from build123d import *

# Parameters (mm, degrees)
BOSS_EXTRUDE1_DEPTH = 5
SKETCH4_R           = 1.75
CUT_EXTRUDE1_DEPTH  = 5
CUT_EXTRUDE2_DEPTH  = 5
SKETCH6_R           = 1.75
BOSS_EXTRUDE2_DEPTH = 5
SKETCH7_W           = 65
SKETCH7_H           = 7
CUT_EXTRUDE3_DEPTH  = 10
FILLET1_R           = 6
FILLET2_R           = 2.5


with BuildPart() as part:
    # Sketch3 → Boss-Extrude1 (new body)
    with BuildSketch(Plane(origin=(0, 0, 0), x_dir=(1, 0, 0), z_dir=(0, 1, 0))):
        Polygon((-32.5, 12), (-32.5, 22), (-22.5, 22), (22.5, 22), (32.5, 22), (32.5, 12), (32.5, 0), (-32.5, 0), align=None)
    extrude(amount=BOSS_EXTRUDE1_DEPTH)

    # Sketch4 → Cut-Extrude1 (cut)
    with BuildSketch(Plane(origin=(0, 5, 0), x_dir=(1, 0, 0), z_dir=(0, 1, 0))):
        with Locations(Location((-25, 5, 0), (0, 0, 270))):
            Circle(SKETCH4_R)
        with Locations(Location((0, 15.5, 0), (0, 0, 270))):
            Circle(SKETCH4_R)
        with Locations(Location((25, 5, 0), (0, 0, 270))):
            Circle(SKETCH4_R)
        with BuildLine():
            Line((-17.5, 0), (17.5, 0))
            Line((17.5, 0), (17.5, 2.5))
            ThreePointArc((17.5, 2.5), (15.596194078, 7.096194078), (11, 9))
            Line((11, 9), (-11, 9))
            ThreePointArc((-11, 9), (-15.596194078, 7.096194078), (-17.5, 2.5))
            Line((-17.5, 2.5), (-17.5, 0))
        make_face()
    extrude(amount=-CUT_EXTRUDE1_DEPTH, mode=Mode.SUBTRACT)

    # Sketch5 → Cut-Extrude2 (cut)
    with BuildSketch(Plane(origin=(0, 5, 0), x_dir=(1, 0, 0), z_dir=(0, 1, 0))):
        with BuildLine():
            Line((-26.75, 5), (-26.75, 8))
            ThreePointArc((-26.75, 8), (-25, 9.75), (-23.25, 8))
            Line((-23.25, 8), (-23.25, 5))
            Line((-23.25, 5), (-26.75, 5))
        make_face()
        with BuildLine():
            Line((23.25, 5), (26.75, 5))
            Line((26.75, 5), (26.75, 8.5))
            ThreePointArc((26.75, 8.5), (25, 10.25), (23.25, 8.5))
            Line((23.25, 8.5), (23.25, 5))
        make_face()
    extrude(amount=-CUT_EXTRUDE2_DEPTH, mode=Mode.SUBTRACT)

    # Sketch6 → Boss-Extrude2 (add)
    with BuildSketch(Plane(origin=(0, 5, 0), x_dir=(1, 0, 0), z_dir=(0, 1, 0))):
        with Locations((0, 15.5)):
            Circle(SKETCH6_R)
    extrude(amount=-BOSS_EXTRUDE2_DEPTH)

    # Sketch7 → Cut-Extrude3 (cut)
    with BuildSketch(Plane(origin=(0, 5, 0), x_dir=(1, 0, 0), z_dir=(0, 1, 0))):
        with Locations((0, 18.5)):
            Rectangle(SKETCH7_W, SKETCH7_H)
    extrude(amount=-CUT_EXTRUDE3_DEPTH, mode=Mode.SUBTRACT)

    # Fillet1
    fillet1_edges = [part.edges().sort_by_distance(p)[0] for p in [
        (-32.5, 2.5, -15),
        (32.5, 2.5, -15),
    ]]
    fillet(fillet1_edges, radius=FILLET1_R)

    # Fillet2
    fillet2_edges = [part.edges().sort_by_distance(p)[0] for p in [
        (0, 5, -15),
        (-32.5, 5, -4.5),
        (-30.742640687, 5, -13.242640687),
        (30.742640687, 5, -13.242640687),
        (32.5, 5, -4.5),
    ]]
    fillet(fillet2_edges, radius=FILLET2_R)


solid = part.part
Model file for the job. Use its own axes, mm. A direction names the side the tool comes from. Give positions to 0.01 mm unless a question says otherwise; leave off trailing zeros. Loops run counter-clockwise (first coordinate to the right, second up) from the corner with the lowest first, then second, coordinate; pieces in that order, holes last.
1) Saw through at A-A (z = -1.5). Write the cut outline in (x, y), plus the area to 3 significant figures.
2) Flat gauge pins, fed straight in: pin 1 Ø1.5 at (y, z) = (4, -11.5) entering from +X; pin 2 Ø1 at (y, z) = (4, -2.5) entering from +X. Where does each tip first touch, or does it go through?
3) Saw through at D-D (x = -25). Write the cut outline in (y, z), plus the area to 3 significant figures.
4) Saw through at C-C (y = 0.6). Write the cut outline in (x, z).
5) Wall check: line 1 (X direction, y = 1.2, z = -1.25); line 2 (X direction, y = 3.85, z = -5.75); line 3 (X direction, y = 3, z = -8). Give the ranges that are in metal, low to high.
6) Tool access for faces 5 (the flat face through (0, 3, -9)), 6 (the cylindrical face through (0.371, 4.287, -14.248)), 7 (the cylindrical face through (25.04, 2.54, -10.25)): list every direction of +Z, -Z, +X, -X, +Y, -Y with a clear straight run to the whole face (end or side of a thin tool).
7) Saw through at B-B (x = 25). Write the cut outline in (y, z).
8) Pull direction Z, two halves, no side cores. Call faces 1 (the flat face through (26.75, 3, -7)), 2 (the cylindrical face through (-15.545, 2.535, -7.146)), 3 (the cylindrical face through (-30.696, 1.232, -13.289)), 4 (the flat face through (-26.75, 3, -6)): +Z half, -Z half, draft (parallel to the pull), parting line (faces both ways), or undercut.
Answer block:
1. outline: (-32.5, 0) - (-17.5, 0) - (-17.5, 5) - (-30, 5) arc R2.5 ccw to (-32.5, 2.5) - close; (17.5, 0) - (32.5, 0) - (32.5, 2.5) arc R2.5 ccw to (30, 5) - (17.5, 5) - close
1. area: 147 mm2
2. pin 1: stops at x = 31.96
2. pin 2: stops at x = 32.29
3. outline: (0, -15) - (2.5, -15) arc R2.5 ccw to (5, -12.5) - (5, -9.75) - (0, -9.75) - close; (0, -3.25) - (5, -3.25) - (5, 0) - (0, 0) - close
3. area: 41.2 mm2
4. outline: (-32.5, -9) arc R6 ccw to (-26.5, -15) - (26.5, -15) arc R6 ccw to (32.5, -9) - (32.5, 0) - (17.5, 0) - (17.5, -2.5) arc R6.5 cw to (11, -9) - (-11, -9) arc R6.5 cw to (-17.5, -2.5) - (-17.5, 0) - (-32.5, 0) - close; hole (-26.75, -8) arc R1.75 ccw to (-23.25, -8) - (-23.25, -5) arc R1.75 ccw to (-26.75, -5) - close; hole (23.25, -8.5) arc R1.75 ccw to (26.75, -8.5) - (26.75, -5) arc R1.75 ccw to (23.25, -5) - close
5. line 1: x = -32.5 to -17.5, 17.5 to 32.5
5. line 2: x = -32.1 to -26.75, -23.25 to -16.63, 16.63 to 23.25, 26.75 to 32.1
5. line 3: x = -32.45 to -26.75, -23.25 to -14.46, 14.46 to 23.25, 26.75 to 32.45
6. face 5: +Z, +Y, -Y
6. face 6: -Z, +X, -X, +Y
6. face 7: +Y, -Y
7. outline: (0, -15) - (2.5, -15) arc R2.5 ccw to (5, -12.5) - (5, -10.25) - (0, -10.25) - close; (0, -3.25) - (5, -3.25) - (5, 0) - (0, 0) - close
8. face 1: undercut
8. face 2: +Z half
8. face 3: -Z half
8. face 4: undercut
